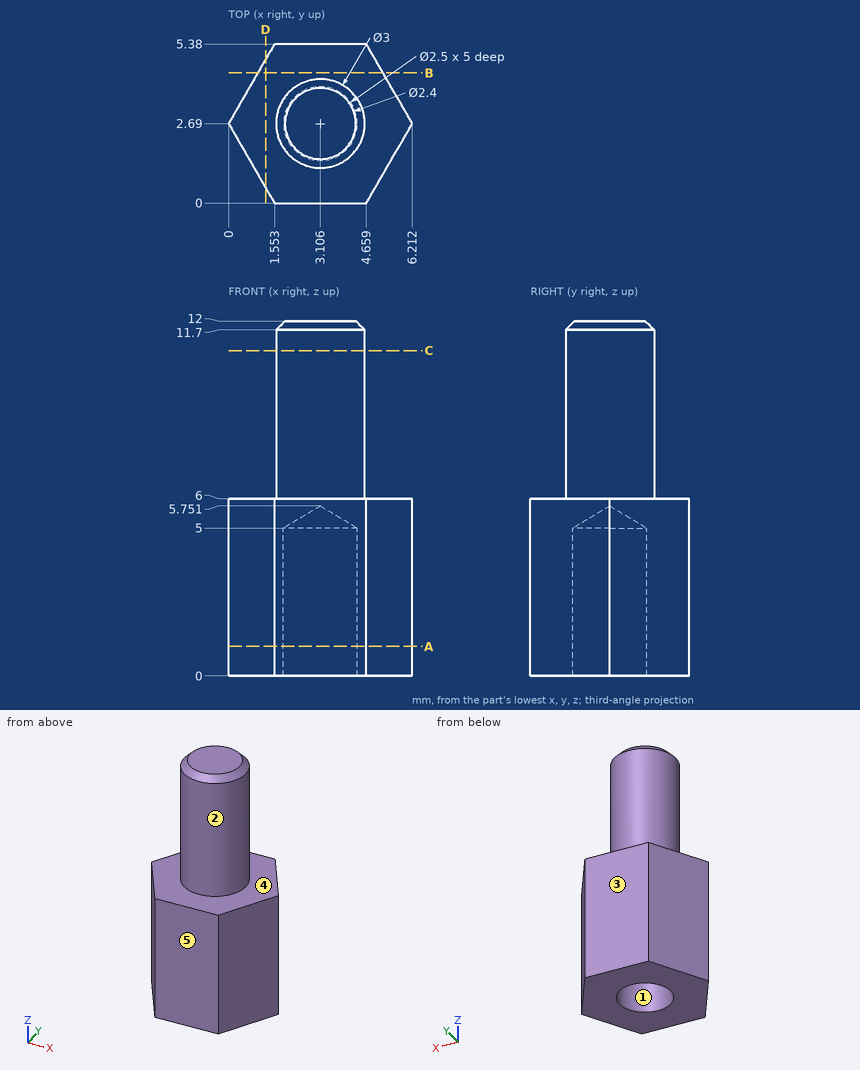
Study the drawing (mm; zero at the part's minimum x, y, z) and answer. A direction names the side the tool comes from. Give positions to 0.01 mm unless a question says otherwise; leave off trailing zeros. Write each loop counter-clockwise with the first axis right and the second up, starting at its lowest first coordinate (ties: lowest second). Pieces come first, ordered by that corner, then holes. Notation, with made-up numbers: (16.25, 54) -> (40.25, 54) arc R7 cw to (40.25, 65) -> close; hole circle Ø4 at (65, 19). An arc over 180 degrees is marked (long way). Answer as a JSON object with one key per item and string values. Group by question number.
1) Find section C-C (z = 11). Write down the section's boundary in (x, y).
2) Find section B-B (y = 4.4). Write down the section's boundary in (x, z) (1 decimal), and give its area (3 significant figures).
3) Find section D-D (x = 1.25). Write down the section's boundary in (y, z) (1 decimal), and give its area (3 significant figures).
4) Find section A-A (z = 1). Write down the section's boundary in (x, y).
5) A tool of negligible diameter and unlimited length cuts with its end or side. For the marked faces 4 and 5, from which of +Z, -Z, +X, -X, +Y, -Y can it reach the whole face along a straight path? Write none if from no direction.
6) This flat-tipped pin is pushed along its axis until it touches: P1, Ø2, axis at y = 4, z = 8.5, coming from the -X side. Where does it stop, or does it pass through?
7) Consider L1, parallel to Z at x = 5.75, y = 3.2; L2, parallel to Y at x = 3.25, z = 3; L3, parallel to X at y = 2.3, z = 2.25 (1 decimal). Determine where each line is inside the solid, lowest interval first. Write a range as from..to.
8) The mould has two halves that part along X. Classify the marked faces 1, 2 and 3: +X half, -X half, draft (parallel to the pull), parting line (faces both ways), or undercut.
Values follow:
{
 "1": {"outline": "circle Ø3 at (3.11, 2.69)"},
 "2": {"outline": "(1, 0) -> (5.2, 0) -> (5.2, 6) -> (1, 6) -> close", "area": "25.4 mm2"},
 "3": {"outline": "(0.5, 0) -> (4.9, 0) -> (4.9, 6) -> (0.5, 6) -> close", "area": "26.0 mm2"},
 "4": {"outline": "(0, 2.69) -> (1.55, 0) -> (4.66, 0) -> (6.21, 2.69) -> (4.66, 5.38) -> (1.55, 5.38) -> close; hole circle Ø2.5 at (3.11, 2.69)"},
 "5": {"face 4": "+Z", "face 5": "+Z, -Z, +X, -X, -Y"},
 "6": {"P1": "stops at x = 1.64"},
 "7": {"L1": "z = 0..6", "L2": "y = 0..1.45, 3.93..5.38", "L3": "x = 0.2..1.9, 4.3..6"},
 "8": {"face 1": "undercut", "face 2": "parting line", "face 3": "draft"}
}
